from build123d import *

# Parameters (mm, degrees)
SKETCH2_R           = 1.7526
BOSS_EXTRUDE1_DEPTH = 5.842
CUT_EXTRUDE1_DEPTH  = 47.691513729


with BuildPart() as part:
    # Sketch2 → Boss-Extrude1 (new body)
    with BuildSketch(Plane.XY.offset(2.794)):
        with BuildLine():
            Line((-0.928725161, 6.398554929), (28.242391074, 13.419823287))
            ThreePointArc((28.242391074, 13.419823287), (39.290541517, 11.000821605), (44.22775, 0.8255))
            ThreePointArc((44.22775, 0.8255), (41.05275, -2.3495), (37.87775, 0.8255))
            ThreePointArc((37.87775, 0.8255), (31.27375, 7.4295), (24.66975, 0.8255))
            Line((24.66975, 0.8255), (24.66975, -1.42875))
            Line((24.66975, -1.42875), (0, -1.42875))
            ThreePointArc((0, -1.42875), (-3.941104949, 2.072380128), (-0.928725161, 6.398554929))
        make_face()
        with Locations((0, 2.54)):
            Circle(SKETCH2_R, mode=Mode.SUBTRACT)
        with Locations((41.05275, 0.8255)):
            Circle(SKETCH2_R, mode=Mode.SUBTRACT)
    extrude(amount=BOSS_EXTRUDE1_DEPTH)

    # Sketch3 → Cut-Extrude1 (cut, through all)
    with BuildSketch(Plane.XY.offset(8.636)):
        with BuildLine():
            Line((37.87775, -10.052724244), (37.87775, 0.8255))
            ThreePointArc((37.87775, 0.8255), (35.220394868, 6.120479725), (29.386892857, 7.154211253))
            Line((29.386892857, 7.154211253), (20.406178571, 4.476679569))
            ThreePointArc((20.406178571, 4.476679569), (18.439954005, 3.102410501), (17.68475, 0.8255))
            Line((17.68475, 0.8255), (17.68475, -10.052724244))
            Line((17.68475, -10.052724244), (37.87775, -10.052724244))
        make_face()
    extrude(amount=-CUT_EXTRUDE1_DEPTH, mode=Mode.SUBTRACT)


solid = part.part
Input: part model. Units: mm. Frame: model coordinates. A direction names the side the tool comes from. Coordinates: 2 decimals unless noted, no trailing zeros. Write each loop counter-clockwise with the first axis right and the second up, starting at its lowest first coordinate (ties: lowest second). Pieces come first, ordered by that corner, then holes. Notation, with made-up numbers: M 88.5,45 L 121.5,45 A14 ccw 121.5,68 Z; hole C -34,33.25 d9. An arc over 180 degrees is marked long. Answer as a JSON object with one key per item and string values. Group by question number.
(1) Section D-D on y = 8. Output: boundary loops of the cut face in (x, z).
(2) Ray query, line 1 along X through (y, z) = (3.75, 6.45); line 2 along X through (y, z) = (3, 3.8); line 3 along Y through (x, z) = (-1.5, 4.45). Return the intervals inside material, ascending. Write a range as [from, to].
(3) Set-up query: faces 1 (the face through (24.959, 5.834, 5.756)), 2 (the face through (9, -1.429, 6)), 3 (the face through (42.67, 0.15, 5.67)). Return all of +Z, -Z, +X, -X, +Y, -Y with unobstructed straight access to the full face (end or side cutting, diameter ignored); none if empty.
(4) Section B-B on y = 1.75. Output: boundary loops of the cut face in (x, z).
(5) Mould query, pull axis X, two halves, no side actions, for faces 4 (the face through (17.685, 0, 6)), 5 (the face through (-3.93, 1.99, 5.67)), 6 (the face through (20, 6, 8.636)). Classes: pulls with the +X half, pulls with the -X half, needs draft (parallel to the pull), parting line crosses it, or undercut.
(6) Section C-C on x = 23.5. Output: boundary loops of the cut face in (y, z).
(7) Section A-A on z = 6.55. Give the number of separate pieces and of enclosed holes in the cut face, plus the area to 3 significant figures.
(8) Contact query for flat-ended pins moving along their axis: P1, Ø3, axis at x = 8, z = 6.5, coming from the -Y side; P2, Ø1.8, axis at y = -0.5, z = 4.5, coming from the +X side; P3, Ø1, axis at x = 4, z = 7.5, coming from the +Y side. Output: stop coordinate, or through.
Result set:
{
 "1": {"outline": "M 5.72,2.79 L 42.06,2.79 L 42.06,8.64 L 5.72,8.64 Z"},
 "2": {"line 1": "x = [-3.78, -1.27], [1.27, 19.05], [37.19, 43.89]", "line 2": "x = [-3.94, -1.69], [1.69, 18.37], [37.51, 44.04]", "line 3": "y = [-1.13, 1.63], [3.45, 6.21]"},
 "3": {"face 1": "+Z, -Z, -Y", "face 2": "+Z, -Z, -X, -Y", "face 3": "+Z, -Z"},
 "4": {"outline": "M -3.89,2.79 L -1.56,2.79 L -1.56,8.64 L -3.89,8.64 Z; M 1.56,2.79 L 17.8,2.79 L 17.8,8.64 L 1.56,8.64 Z; M 37.81,2.79 L 39.56,2.79 L 39.56,8.64 L 37.81,8.64 Z; M 42.54,2.79 L 44.19,2.79 L 44.19,8.64 L 42.54,8.64 Z"},
 "5": {"face 4": "undercut", "face 5": "pulls with the -X half", "face 6": "needs draft"},
 "6": {"outline": "M 5.4,2.79 L 12.28,2.79 L 12.28,8.64 L 5.4,8.64 Z"},
 "7": {"separate pieces": "1", "enclosed holes": "2", "area": "393 mm2"},
 "8": {"P1": "stops at y = -1.43", "P2": "stops at x = 44.2", "P3": "stops at y = 7.71"}
}
